```python
from build123d import *

# Parameters (mm, degrees)
SKETCH1_W           = 31.85
SKETCH1_H           = 7.85
BOSS_EXTRUDE1_DEPTH = 3.2
SKETCH2_R           = 2.45
BOSS_EXTRUDE2_DEPTH = 1.9
SHELL1_T            = -1.5
SKETCH3_R           = 1.5
SKETCH3_R_2         = 0.53
BOSS_EXTRUDE3_DEPTH = 1.5


with BuildPart() as part:
    # Sketch1 → Boss-Extrude1 (new body)
    with BuildSketch(Plane(origin=(0, 0, 0), x_dir=(1, 0, 0), z_dir=(0, 1, 0))):
        Rectangle(SKETCH1_W, SKETCH1_H)
    extrude(amount=-BOSS_EXTRUDE1_DEPTH)

    # Sketch2 → Boss-Extrude2 (add)
    with BuildSketch(Plane(origin=(0, 0, 0), x_dir=(1, 0, 0), z_dir=(0, 1, 0))):
        with Locations(Location((11.94375, 0, 0), (0, 0, 90))):
            Circle(SKETCH2_R)
        with Locations(Location((-11.94375, 0, 0), (0, 0, 90))):
            Circle(SKETCH2_R)
    extrude(amount=BOSS_EXTRUDE2_DEPTH)

    # Shell1
    shell1_openings = [part.faces().sort_by_distance(p)[0] for p in [
        (0, -3.2, 0),
    ]]
    offset(amount=SHELL1_T, openings=shell1_openings, kind=Kind.INTERSECTION)

    # Sketch3 → Boss-Extrude3 (add)
    # profile 1 of 3: a face of its own
    with BuildSketch(Plane.XZ.offset(1.5)):
        with Locations(Location((-7.9625, 0, 0), (0, 0, 90))):
            Circle(SKETCH3_R)
        with Locations(Location((-7.9625, 0, 0), (0, 0, 90))):
            Circle(SKETCH3_R_2, mode=Mode.SUBTRACT)
    # profile 2 of 3: a face of its own
    with BuildSketch(Plane.XZ.offset(1.5)):
        with Locations(Location((0, 0, 0), (0, 0, 90))):
            Circle(SKETCH3_R)
        with Locations(Location((0, 0, 0), (0, 0, 90))):
            Circle(SKETCH3_R_2, mode=Mode.SUBTRACT)
    # profile 3 of 3: a face of its own
    with BuildSketch(Plane.XZ.offset(1.5)):
        with Locations(Location((7.9625, 0, 0), (0, 0, 90))):
            Circle(SKETCH3_R)
        with Locations(Location((7.9625, 0, 0), (0, 0, 90))):
            Circle(SKETCH3_R_2, mode=Mode.SUBTRACT)
    extrude(amount=BOSS_EXTRUDE3_DEPTH)


solid = part.part
```
The listing builds one solid part. Answer for the finished solid, in the listing's coordinates (mm). A direction names the side the tool comes from. Give positions to 0.01 mm unless a question says otherwise; leave off trailing zeros. Order: outer loops, then holes, each group sorted by start corner. A loop starts at its lowest first (then second) coordinate and runs counter-clockwise, first axis right, second up.
1) Determine the mould class of faces 1 (the face through (0, 0, 0)), 2 (the face through (-9.55, 0.94, 0.53)), 3 (the face through (8, -1.5, 0)), 4 (the face through (0, -2, -3.925)) for opening direction Z: pulls with the +Z half, pulls with the -Z half, needs draft (parallel to the pull), parting line crosses it, or undercut.
Reported:
face 1: needs draft
face 2: parting line crosses it
face 3: undercut
face 4: pulls with the -Z half
2) For faces 5 (the face through (-9.45, -2.24, -0.2)), 6 (the face through (12, 1.9, 0)), determine the directions among +Z, -Z, +X, -X, +Y, -Y from which every point of the face is accessible in a straight line to the end or side of a thin tool.
Reported:
face 5: -Y
face 6: +Z, -Z, +X, -X, +Y
3) Find section A-A on y = -2.2. Write down the section's boundary in (x, z) (1 decimal), then the cut area to 3 significant figures.
Reported:
outline: (-15.9, -3.9) - (15.9, -3.9) - (15.9, 3.9) - (-15.9, 3.9) - close; circle Ø3 at (-8, 0); circle Ø3 at (0, 0); circle Ø3 at (8, 0); hole (-14.4, -2.4) - (14.4, -2.4) - (14.4, 2.4) - (-14.4, 2.4) - close; hole circle Ø1.1 at (-8, 0); hole circle Ø1.1 at (0, 0); hole circle Ø1.1 at (8, 0)
area: 129 mm2
4) Consider line 1 along X through (y, z) = (-0.15, 0) (3 decimals); line 2 along Z through (x, y) = (-5.5, -2.9) (3 decimals); line 3 along Y through (x, z) = (12.5, 2.75). Determine where each line is inside the solid, lowest interval first.
Reported:
line 1: x = -15.925 to -12.894, -10.994 to 10.994, 12.894 to 15.925
line 2: z = -3.925 to -2.425, 2.425 to 3.925
line 3: y = -3.2 to 0
5) Find section C-C on y = 1.2. Write down the section's boundary in (x, z).
Reported:
outline: circle Ø4.9 at (-11.94, 0); circle Ø4.9 at (11.94, 0)
6) Find section B-B on x = 0. Write down the section's boundary in (y, z) (3 decimals).
Reported:
outline: (-3.2, -3.925) - (0, -3.925) - (0, 3.925) - (-3.2, 3.925) - (-3.2, 2.425) - (-1.5, 2.425) - (-1.5, 1.5) - (-3, 1.5) - (-3, 0.53) - (-1.5, 0.53) - (-1.5, -0.53) - (-3, -0.53) - (-3, -1.5) - (-1.5, -1.5) - (-1.5, -2.425) - (-3.2, -2.425) - close
7) Given P1, Ø0.6, axis at x = -7.96, z = 0, coming from the -Y side; P2, Ø1.2, axis at x = 0, z = -0.5, coming from the -Y side; P3, Ø1, axis at x = 7.96, z = 0, coming from the +Y side, each flat-ended and moving along its own axis, determine where each tip first touches the part or whether it passes through.
Reported:
P1: stops at y = -1.5
P2: stops at y = -3
P3: stops at y = 0
8) Find section D-D on y = -0.3. Write down the section's boundary in (x, z) (3 decimals), then the cut area to 3 significant figures.
Reported:
outline: (-15.925, -3.925) - (15.925, -3.925) - (15.925, 3.925) - (-15.925, 3.925) - close; hole circle Ø1.9 at (-11.944, 0); hole circle Ø1.9 at (11.944, 0)
area: 244 mm2
